from build123d import *

# Parameters (mm, degrees)
ESBO_O1_W             = 154
ESBO_O1_H             = 69.55
FLANGE_BASE1_DEPTH    = 7.4
ESBO_O6_R             = 4.775
CORTE_EXTRUS_O1_DEPTH = 5.75
ESBO_O8_R             = 2.65
CORTE_EXTRUS_O3_DEPTH = 85.683901215
ESBO_O10_R            = 2.1
CORTE_EXTRUS_O4_DEPTH = 85.811913226


# Sheet-metal steps are written as plain solids
with BuildPart() as part:
    # Esboço1 → Flange-base1 (new body)
    with BuildSketch(Plane(origin=(0, 0, 0), x_dir=(1, 0, 0), z_dir=(0, 1, 0))):
        Rectangle(ESBO_O1_W, ESBO_O1_H)
    extrude(amount=-FLANGE_BASE1_DEPTH)

    # Esboço6 → Corte-extrusão1 (cut)
    with BuildSketch(Plane(origin=(0, 0, 0), x_dir=(1, 0, 0), z_dir=(0, 1, 0))):
        with Locations(Location((-50, 13, 0), (0, 0, 270))):
            Circle(ESBO_O6_R)
        with Locations(Location((-50, -13, 0), (0, 0, 270))):
            Circle(ESBO_O6_R)
        with Locations(Location((-12, 15, 0), (0, 0, 270))):
            Circle(ESBO_O6_R)
        with Locations(Location((12, 15, 0), (0, 0, 270))):
            Circle(ESBO_O6_R)
        with Locations(Location((12, -15, 0), (0, 0, 270))):
            Circle(ESBO_O6_R)
        with Locations(Location((50, 13, 0), (0, 0, 270))):
            Circle(ESBO_O6_R)
        with Locations(Location((50, -13, 0), (0, 0, 270))):
            Circle(ESBO_O6_R)
        with Locations(Location((-12, -15, 0), (0, 0, 270))):
            Circle(ESBO_O6_R)
    extrude(amount=-CORTE_EXTRUS_O1_DEPTH, mode=Mode.SUBTRACT)

    # Esboço8 → Corte-extrusão3 (cut, through all)
    with BuildSketch(Plane(origin=(0, -5.75, 0), x_dir=(1, 0, 0), z_dir=(0, 1, 0))):
        with Locations(Location((-50, 13, 0), (0, 0, 270))):
            Circle(ESBO_O8_R)
        with Locations(Location((-50, -13, 0), (0, 0, 270))):
            Circle(ESBO_O8_R)
        with Locations(Location((-12, 15, 0), (0, 0, 270))):
            Circle(ESBO_O8_R)
        with Locations(Location((12, 15, 0), (0, 0, 270))):
            Circle(ESBO_O8_R)
        with Locations(Location((12, -15, 0), (0, 0, 270))):
            Circle(ESBO_O8_R)
        with Locations(Location((50, 13, 0), (0, 0, 270))):
            Circle(ESBO_O8_R)
        with Locations(Location((50, -13, 0), (0, 0, 270))):
            Circle(ESBO_O8_R)
        with Locations(Location((-12, -15, 0), (0, 0, 270))):
            Circle(ESBO_O8_R)
    extrude(amount=-CORTE_EXTRUS_O3_DEPTH, mode=Mode.SUBTRACT)

    # Esboço10 → Corte-extrusão4 (cut, through all)
    with BuildSketch(Plane(origin=(0, 0, 0), x_dir=(1, 0, 0), z_dir=(0, 1, 0))):
        with Locations(Location((-67, 13.626456062, 0), (0, 0, 270))):
            Circle(ESBO_O10_R)
        with Locations(Location((-67, -12.373543938, 0), (0, 0, 270))):
            Circle(ESBO_O10_R)
        with Locations(Location((67, 13, 0), (0, 0, 270))):
            Circle(ESBO_O10_R)
        with Locations(Location((67, -13, 0), (0, 0, 270))):
            Circle(ESBO_O10_R)
    extrude(amount=-CORTE_EXTRUS_O4_DEPTH, mode=Mode.SUBTRACT)


solid = part.part
Check sheet for the modelled part. Datum: model origin and axes. Units: mm. A direction names the side the tool comes from. Give positions to 0.01 mm unless a question says otherwise; leave off trailing zeros. Order: outer loops, then holes, each group sorted by start corner. A loop starts at its lowest first (then second) coordinate and runs counter-clockwise, first axis right, second up. Notation, with made-up numbers: M -38.75,45 L -4.75,45 A19 cw -4.75,61 Z; hole C 38.25,-24.5 d5. An arc over 180 degrees is marked long. Answer as CSV lines item,"result". Start each with the question number.
Item 1: Cross-section at B-B on y = -3.75. State how many separate pieces and enclosed holes the cut face has, plus the area to 3 significant figures.
Item 2: Gauge pin test, flat end, axial feed: P1, Ø5.5, axis at x = -50, z = 13, coming from the +Y side. Record the tip position at first contact, or that the pin passes through.
Item 3: Thickness scan on line 1 (Z direction, x = -10, y = -3.75) (3 decimals); line 2 (Y direction, x = -16, z = -17). Record the ranges inside material, lowest first. Write a range as [from, to].
Item 4: Cross-section at A-A on x = 67. Enter the section's corners in (y, z) (3 decimals), plus the area to 3 significant figures.
Item 5: Tool access check on faces 4 (the face through (10, -5.75, -13)), 5 (the face through (65.722, -3.648, 11.334)). Record the directions out of +Z, -Z, +X, -X, +Y, -Y that give a thin tool (end or side, any length) a straight path to the whole face; none if there is none.
Item 6: Mould release check, pull along Z, two halves, no side actions. Record for faces 1 (the face through (-1, -4, -34.775)), 2 (the face through (51.434, -2.835, 17.554)), 3 (the face through (-77, -4, 0)): +Z half, -Z half, draft (parallel to the pull), parting line (faces both ways), or undercut.
Item 7: Cross-section at C-C on x = -12. Enter the section's corners in (y, z) (3 decimals).
Established:
1,separate pieces,"1"
1,enclosed holes,"12"
1,area,"10,100 mm^2"
2,P1,"stops at y = -5.75"
3,line 1,"z = [-34.775, -19.336], [-10.664, 10.664], [19.336, 34.775]"
3,line 2,"y = [-7.4, -5.75]"
4,outline,"M -7.4,-34.775 L 0,-34.775 L 0,-15.1 L -7.4,-15.1 Z; M -7.4,-10.9 L 0,-10.9 L 0,10.9 L -7.4,10.9 Z; M -7.4,15.1 L 0,15.1 L 0,34.775 L -7.4,34.775 Z"
4,area,"453 mm^2"
5,face 4,"+Y"
5,face 5,"+Y, -Y"
6,face 1,"-Z half"
6,face 2,"undercut"
6,face 3,"draft"
7,outline,"M -7.4,-34.775 L 0,-34.775 L 0,-19.775 L -5.75,-19.775 L -5.75,-17.65 L -7.4,-17.65 Z; M -7.4,-12.35 L -5.75,-12.35 L -5.75,-10.225 L 0,-10.225 L 0,10.225 L -5.75,10.225 L -5.75,12.35 L -7.4,12.35 Z; M -7.4,17.65 L -5.75,17.65 L -5.75,19.775 L 0,19.775 L 0,34.775 L -7.4,34.775 Z"
